The drawing under review shows one solid part. Ordinate dimensions are in mm from its lowest x, y, z. A direction names the side the tool comes from. Give positions to 0.01 mm unless a question says otherwise; leave off trailing zeros. Order: outer loops, then holes, each group sorted by start corner. A loop starts at its lowest first (then second) coordinate and runs counter-clockwise, first axis right, second up. Notation, with made-up numbers: (30.25, -10.75) - (83.25, -10.75) arc R33 ccw to (83.25, 20.25) - close; hole circle Ø11 at (35.5, -36). An arc over 180 degrees is marked (long way). Use CSV: the item, a comma, the result in double quotes. Start each with the question number.
1. Draft analysis for pull direction X (two halves, no side actions). For the marked faces 3, 4 and 5, state which applies: released by +X, released by -X, zero draft, split by the parting line, or undercut.
2. Take a section at B-B, the plane x = 17.5. State the section outline as (y, z) points, then the cut area to 3 significant figures.
3. Take a section at D-D, the plane z = 6. State the section outline as (x, y) points, then the cut area to 3 significant figures.
4. Take a section at A-A, the plane z = 4. State the section outline as (x, y) points, then the cut area to 4 significant figures.
5. Take a section at C-C, the plane x = 38.5. State the section outline as (y, z) points, then the cut area to 3 significant figures.
6. Machinability: for the marked faces 1 and 2, which of the approach directions +Z, -Z, +X, -X, +Y, -Y give a long, thin tool a straight path to every point of the face, cutting with its end or side? Answer none if there is none.
7. To check wall thickness, follow line 1 (Y direction, x = 38.5, z = 1.5); line 2 (Y direction, x = 40, z = 1.5); line 3 (Y direction, x = 24.5, z = 3.25). State the ranges of each line that lie inside material, in increasing order. Write a range as [from, to].
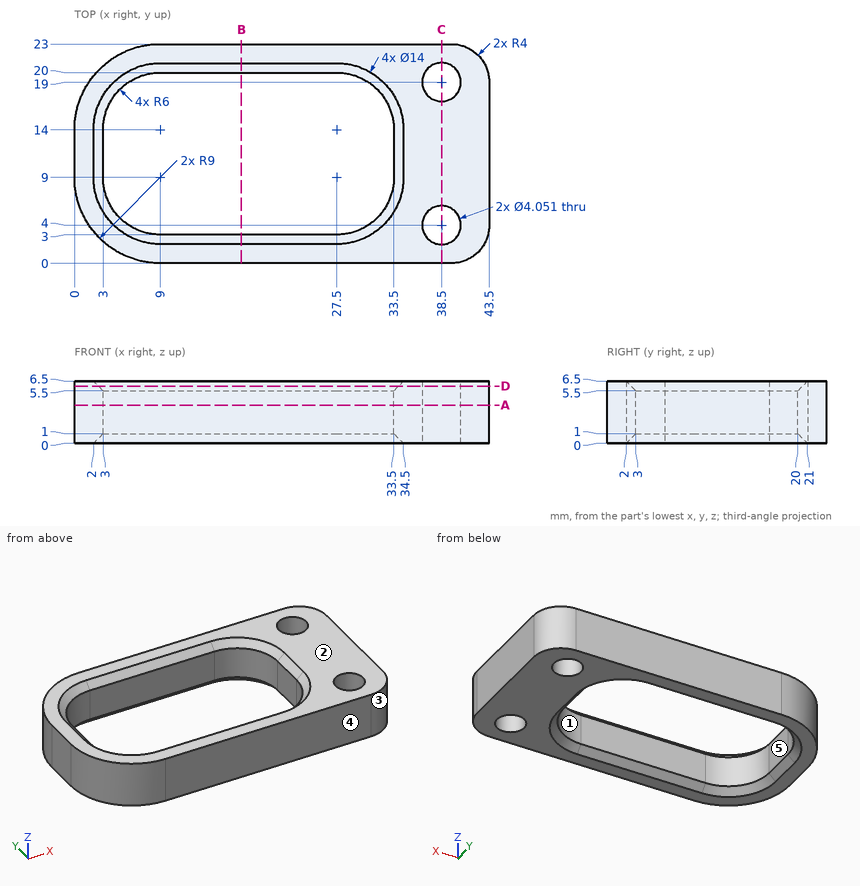
Determined:
1,face 3,"released by +X"
1,face 4,"zero draft"
1,face 5,"undercut"
2,outline,"(0, 0) - (2, 0) - (3, 1) - (3, 5.5) - (2, 6.5) - (0, 6.5) - close; (20, 1) - (21, 0) - (23, 0) - (23, 6.5) - (21, 6.5) - (20, 5.5) - close"
2,area,"37.0 mm²"
3,outline,"(0, 9) arc R9 ccw to (9, 0) - (39.5, 0) arc R4 ccw to (43.5, 4) - (43.5, 19) arc R4 ccw to (39.5, 23) - (9, 23) arc R9 ccw to (0, 14) - close; hole (2.5, 9) arc R6.5 ccw to (9, 2.5) - (27.5, 2.5) arc R6.5 ccw to (34, 9) - (34, 14) arc R6.5 ccw to (27.5, 20.5) - (9, 20.5) arc R6.5 ccw to (2.5, 14) - close; hole circle Ø4.05 at (38.5, 4); hole circle Ø4.05 at (38.5, 19)"
3,area,"402 mm²"
4,outline,"(0, 9) arc R9 ccw to (9, 0) - (39.5, 0) arc R4 ccw to (43.5, 4) - (43.5, 19) arc R4 ccw to (39.5, 23) - (9, 23) arc R9 ccw to (0, 14) - close; hole (3, 9) arc R6 ccw to (9, 3) - (27.5, 3) arc R6 ccw to (33.5, 9) - (33.5, 14) arc R6 ccw to (27.5, 20) - (9, 20) arc R6 ccw to (3, 14) - close; hole circle Ø4.05 at (38.5, 4); hole circle Ø4.05 at (38.5, 19)"
4,area,"445.5 mm²"
5,outline,"(0, 0) - (1.97, 0) - (1.97, 6.5) - (0, 6.5) - close; (6.03, 0) - (16.97, 0) - (16.97, 6.5) - (6.03, 6.5) - close; (21.03, 0) - (23, 0) - (23, 6.5) - (21.03, 6.5) - close"
5,area,"96.8 mm²"
6,face 1,"+Z, -Z"
6,face 2,"+Z, +X, -X, +Y, -Y"
7,line 1,"y = [0, 1.97], [6.03, 16.97], [21.03, 23]"
7,line 2,"y = [0.03, 2.64], [5.36, 17.64], [20.36, 22.97]"
7,line 3,"y = [0, 3], [20, 23]"
